Can you work these out from the model? Positions are in its coordinate system, mm. Coordinates: 2 decimals unless noted, no trailing zeros. Order: outer loops, then holes, each group sorted by start corner. A loop starts at its lowest first (then second) coordinate and runs counter-clockwise, first axis right, second up. Notation, with made-up numbers: (45.25, 84) -> (79.25, 84) arc R35 cw to (79.25, 121) -> close; hole circle Ø4 at (57, 80.25). An arc over 180 degrees is marked (long way). Answer in a Markdown table with one row per item.
```python
from build123d import *

# Parameters (mm, degrees)
SKETCH1_W           = 50
SKETCH1_H           = 25
BOSS_EXTRUDE1_DEPTH = 4
SKETCH1_3_W         = 8
SKETCH1_3_H         = 8
SKETCH1_3_R         = 1.5
SKETCH1_3_R_2       = 3
CUT_EXTRUDE3_DEPTH  = 3
SKETCH1_4_R         = 1.5
SKETCH1_4_R_2       = 3
CUT_EXTRUDE4_DEPTH  = 57.044625077


with BuildPart() as part:
    # Sketch1 → Boss-Extrude1 (new body)
    with BuildSketch(Plane(origin=(0, 0, 0), x_dir=(1, 0, 0), z_dir=(0, 1, 0))):
        with Locations((25, 12.5)):
            Rectangle(SKETCH1_W, SKETCH1_H)
    extrude(amount=BOSS_EXTRUDE1_DEPTH)

    # Sketch1_3 → Cut-Extrude3 (cut)
    # profile 1 of 6: a face of its own
    with BuildSketch(Plane(origin=(0, 0, 0), x_dir=(1, 0, 0), z_dir=(0, 1, 0))):
        with Locations((42, 8)):
            Rectangle(SKETCH1_3_W, SKETCH1_3_H)
        with Locations(Location((42, 8, 0), (0, 0, 270))):
            Circle(SKETCH1_3_R, mode=Mode.SUBTRACT)
    # profile 2 of 6: a face of its own
    with BuildSketch(Plane(origin=(0, 0, 0), x_dir=(1, 0, 0), z_dir=(0, 1, 0))):
        with Locations((42, 17)):
            Rectangle(SKETCH1_3_W, SKETCH1_3_H)
        with Locations(Location((42, 17, 0), (0, 0, 270))):
            Circle(SKETCH1_3_R, mode=Mode.SUBTRACT)
    # profile 3 of 6: a face of its own
    with BuildSketch(Plane(origin=(0, 0, 0), x_dir=(1, 0, 0), z_dir=(0, 1, 0))):
        with Locations((31, 12.5)):
            Rectangle(SKETCH1_3_W, SKETCH1_3_H)
        with Locations(Location((31, 12.5, 0), (0, 0, 270))):
            Circle(SKETCH1_3_R_2, mode=Mode.SUBTRACT)
    # profile 4 of 6: a face of its own
    with BuildSketch(Plane(origin=(0, 0, 0), x_dir=(1, 0, 0), z_dir=(0, 1, 0))):
        with Locations((8, 8)):
            Rectangle(SKETCH1_3_W, SKETCH1_3_H)
        with Locations(Location((8, 8, 0), (0, 0, 270))):
            Circle(SKETCH1_3_R, mode=Mode.SUBTRACT)
    # profile 5 of 6: a face of its own
    with BuildSketch(Plane(origin=(0, 0, 0), x_dir=(1, 0, 0), z_dir=(0, 1, 0))):
        with Locations((19, 12.5)):
            Rectangle(SKETCH1_3_W, SKETCH1_3_H)
    # profile 6 of 6: a face of its own
    with BuildSketch(Plane(origin=(0, 0, 0), x_dir=(1, 0, 0), z_dir=(0, 1, 0))):
        with Locations((8, 17)):
            Rectangle(SKETCH1_3_W, SKETCH1_3_H)
    extrude(amount=CUT_EXTRUDE3_DEPTH, mode=Mode.SUBTRACT)

    # Sketch1_4 → Cut-Extrude4 (cut, through all)
    with BuildSketch(Plane(origin=(0, 0, 0), x_dir=(1, 0, 0), z_dir=(0, 1, 0))):
        with Locations(Location((8, 17, 0), (0, 0, 270))):
            Circle(SKETCH1_4_R)
        with Locations(Location((42, 17, 0), (0, 0, 90))):
            Circle(SKETCH1_4_R)
        with Locations(Location((42, 8, 0), (0, 0, 270))):
            Circle(SKETCH1_4_R)
        with Locations(Location((31, 12.5, 0), (0, 0, 90))):
            Circle(SKETCH1_4_R_2)
        with Locations(Location((19, 12.5, 0), (0, 0, 270))):
            Circle(SKETCH1_4_R_2)
        with Locations(Location((8, 8, 0), (0, 0, 90))):
            Circle(SKETCH1_4_R)
    extrude(amount=CUT_EXTRUDE4_DEPTH, mode=Mode.SUBTRACT)


solid = part.part
```
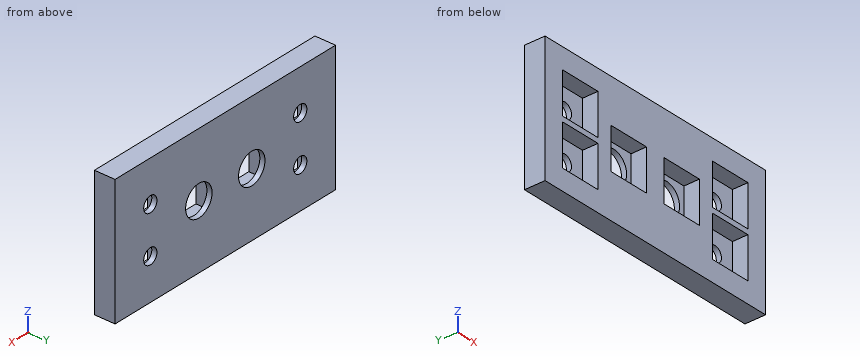
(1) I need wall thicknesses on line 1 (X direction, y = 3.3, z = -12.5); line 2 (Z direction, x = 45, y = 1.7); line 3 (X direction, y = 0.25, z = -17). Which ranges of each line are inside material? Lowest first, please. Write a range as [from, to].
Response values:
| item | result |
|---|---|
| line 1 | [0, 16], [22, 28], [34, 50] |
| line 2 | [-25, -21], [-13, -12], [-4, 0] |
| line 3 | [0, 4], [12, 38], [46, 50] |
(2) Suppose I cut it at C-C (y = 2.15). Please give me the cut outline in (x, z), and give its area (3 significant figures).
Response values:
| item | result |
|---|---|
| outline | (0, -25) -> (50, -25) -> (50, 0) -> (0, 0) -> close; hole (4, -21) -> (12, -21) -> (12, -13) -> (4, -13) -> close; hole (4, -12) -> (12, -12) -> (12, -4) -> (4, -4) -> close; hole (15, -16.5) -> (23, -16.5) -> (23, -8.5) -> (15, -8.5) -> close; hole (27, -16.5) -> (35, -16.5) -> (35, -8.5) -> (27, -8.5) -> close; hole (38, -21) -> (46, -21) -> (46, -13) -> (38, -13) -> close; hole (38, -12) -> (46, -12) -> (46, -4) -> (38, -4) -> close |
| area | 866 mm2 |
(3) Suppose I cut it at D-D (z = -20). Please give me the cut outline in (x, y), and give its area (3 significant figures).
Response values:
| item | result |
|---|---|
| outline | (0, 0) -> (4, 0) -> (4, 3) -> (12, 3) -> (12, 0) -> (38, 0) -> (38, 3) -> (46, 3) -> (46, 0) -> (50, 0) -> (50, 4) -> (0, 4) -> close |
| area | 152 mm2 |
(4) Suppose I cut it at B-B (x = 19). Please give me the cut outline in (y, z), and give its area (3 significant figures).
Response values:
| item | result |
|---|---|
| outline | (0, -25) -> (4, -25) -> (4, -15.5) -> (3, -15.5) -> (3, -16.5) -> (0, -16.5) -> close; (0, -8.5) -> (3, -8.5) -> (3, -9.5) -> (4, -9.5) -> (4, 0) -> (0, 0) -> close |
| area | 70.0 mm2 |
(5) Will these pins go through, and if not, where does the flat tip stop? pin 1 Ø2.5 at (x, z) = (8.5, -9.5) entering from -Y; pin 2 Ø2.5 at (x, z) = (42, -8) entering from -Y.
Response values:
| item | result |
|---|---|
| pin 1 | y = 3 |
| pin 2 | through |
(6) Suppose I cut it at A-A (z = -8). Please give me the cut outline in (x, y), and give its area (3 significant figures).
Response values:
| item | result |
|---|---|
| outline | (0, 0) -> (4, 0) -> (4, 3) -> (6.5, 3) -> (6.5, 4) -> (0, 4) -> close; (9.5, 3) -> (12, 3) -> (12, 0) -> (38, 0) -> (38, 3) -> (40.5, 3) -> (40.5, 4) -> (9.5, 4) -> close; (43.5, 3) -> (46, 3) -> (46, 0) -> (50, 0) -> (50, 4) -> (43.5, 4) -> close |
| area | 146 mm2 |
